Model file for the job. Use its own axes, mm. A direction names the side the tool comes from. Coordinates: 2 decimals unless noted, no trailing zeros. Write each loop counter-clockwise with the first axis right and the second up, starting at its lowest first coordinate (ties: lowest second). Pieces come first, ordered by that corner, then holes.
Q1. Pin check, flat tips, straight feed: P1, Ø3, axis at x = 28.5, y = -37, coming from the -Z side; P2, Ø6, axis at x = 27, z = 31, coming from the -Y side; P3, Ø2, axis at x = 29, y = -1, coming from the +Z side. Stop position of each tip, or through.
Q2. Which spindle directions (+Z, -Z, +X, -X, +Y, -Y) get a long thin tool onto all of the face, cutting with end or side? Do faces 4 (the flat face through (29.892, -54, -40)), 5 (the flat face through (4, 40.028, 66)), 6 (the flat face through (-32, 36.214, -40)), 7 (the flat face through (-24.734, 46, 31)). Say none if no direction does.
Q3. Drill centre lines: probe 1 along X at (y, z) = (43, 42); probe 2 along X at (y, z) = (46, -50.5); probe 3 along Y at (x, z) = (31.5, -57). Where is each one in solid material? Low to high.
Q4. Band-saw the part on C-C, the plane z = 47. Write the cut outline in (x, y), plus the area to 3 significant figures.
Q5. Pull direction Z, two halves, no side cores. Call faces 1 (the flat face through (-25.249, -54, -40)), 2 (the flat face through (39, 44, -81.651)), 3 (the flat face through (32.607, 46, 31)): released by +Z, released by -Z, zero draft, split by the parting line, or undercut.
Q6. Band-saw the part on B-B, the plane x = 7. Write the cut outline in (y, z), plus the area to 3 significant figures.
Q7. Band-saw the part on D-D, the plane y = 43.5. Write the cut outline in (x, z).
Q8. Band-saw the part on A-A, the plane z = -49. Write the cut outline in (x, y).
from build123d import *

# Parameters (mm, degrees)
F0_W     = 86.1037485301
F0_H     = 112.4806329608
F1_DEPTH = 12.7
F2_W     = 13.9083378017
F2_H     = 11.3344117999
F2_W_2   = 14.853797853
F3_DEPTH = 88.5675344616
F4_W     = 17.5688937306
F4_H     = 13.3278891444
F4_H_2   = 15.1476562023
F4_W_2   = 13.3936516941
F5_DEPTH = 71.4913029224
F6_W     = 11.3344117999
F6_H     = 50.6459615797
F7_DEPTH = 57.3416128755
F8_DEPTH = 10.16


with BuildPart() as f1:
    # F0 (on Top) → F1 (new body)
    with BuildSketch(Plane.XY):
        with Locations((4.4093746692, -4.878398031)):
            Rectangle(F0_W, F0_H)
    extrude(amount=F1_DEPTH)

    # F2 (on face) → F3 (join)
    with BuildSketch(Plane.XY.offset(12.7)):
        with Locations((-31.688330695, 45.6947125494)):
            Rectangle(F2_W, F2_H)
        with Locations((40.0343500078, 45.6947125494)):
            Rectangle(F2_W_2, F2_H)
    extrude(amount=F3_DEPTH)

    # F4 (on face) → F5 (join)
    with BuildSketch(Plane(origin=(0, 0, 0), x_dir=(1, 0, 0), z_dir=(0, 0, -1))):
        with Locations((38.6768020689, 54.4547699392)):
            Rectangle(F4_W, F4_H)
        with Locations((38.6768020689, -43.7880903482)):
            Rectangle(F4_W, F4_H_2)
        with Locations((-31.9456737489, -43.7880903482)):
            Rectangle(F4_W_2, F4_H_2)
        with Locations((-31.9456737489, 54.4547699392)):
            Rectangle(F4_W_2, F4_H)
    extrude(amount=F5_DEPTH)

    # F6 (on face) → F7 (join, through all)
    with BuildSketch(Plane.YZ.offset(-24.7341617942)):
        with Locations((45.6947125494, 75.9445536718)):
            Rectangle(F6_W, F6_H)
    extrude(amount=F7_DEPTH)

    # F8 (add): faces of the model
    f8_faces = [f1.faces().sort_by_distance(p)[0] for p in [
        (-31.9456737489, -54.4547699392, -71.4913029224),
        (38.6768020689, -54.4547699392, -71.4913029224),
        (38.6768020689, 43.7880903482, -71.4913029224),
        (-31.9456737489, 43.7880903482, -71.4913029224),
        (-31.9456737489, -54.4547699392, -71.4913029224),
        (38.6768020689, -54.4547699392, -71.4913029224),
        (38.6768020689, 43.7880903482, -71.4913029224),
        (-31.9456737489, 43.7880903482, -71.4913029224),
        (-31.9456737489, -54.4547699392, -71.4913029224),
        (38.6768020689, -54.4547699392, -71.4913029224),
        (38.6768020689, 43.7880903482, -71.4913029224),
        (-31.9456737489, 43.7880903482, -71.4913029224),
        (-31.9456737489, -54.4547699392, -71.4913029224),
        (38.6768020689, -54.4547699392, -71.4913029224),
        (38.6768020689, 43.7880903482, -71.4913029224),
        (-31.9456737489, 43.7880903482, -71.4913029224),
    ]]
    extrude(f8_faces, amount=F8_DEPTH)


solid = f1.part
Answer sheet:
1. P1: stops at z = 0
1. P2: passes through
1. P3: stops at z = 12.7
2. face 4: -Z, +Y, -Y
2. face 5: +Z, +X, -X, -Y
2. face 6: -Z, +X, -X
2. face 7: +Y, -Y
3. probe 1: x = -38.64 to -24.73, 32.61 to 47.46
3. probe 2: x = -38.64 to -25.25, 29.89 to 47.46
3. probe 3: y = -61.12 to -47.79, 36.21 to 51.36
4. outline: (-38.64, 40.03) - (-24.73, 40.03) - (-24.73, 51.36) - (-38.64, 51.36) - close; (32.61, 40.03) - (47.46, 40.03) - (47.46, 51.36) - (32.61, 51.36) - close
4. area: 326 mm2
5. face 1: zero draft
5. face 2: released by -Z
5. face 3: undercut
6. outline: (-61.12, 0) - (51.36, 0) - (51.36, 12.7) - (-61.12, 12.7) - close; (40.03, 50.62) - (51.36, 50.62) - (51.36, 101.27) - (40.03, 101.27) - close
6. area: 2,000 mm2
7. outline: (-38.64, -81.65) - (-25.25, -81.65) - (-25.25, 0) - (29.89, 0) - (29.89, -81.65) - (47.46, -81.65) - (47.46, 101.27) - (-38.64, 101.27) - close; hole (-24.73, 12.7) - (32.61, 12.7) - (32.61, 50.62) - (-24.73, 50.62) - close
8. outline: (-38.64, -61.12) - (-25.25, -61.12) - (-25.25, -47.79) - (-38.64, -47.79) - close; (-38.64, 36.21) - (-25.25, 36.21) - (-25.25, 51.36) - (-38.64, 51.36) - close; (29.89, -61.12) - (47.46, -61.12) - (47.46, -47.79) - (29.89, -47.79) - close; (29.89, 36.21) - (47.46, 36.21) - (47.46, 51.36) - (29.89, 51.36) - close
